```python
from build123d import *

# Parameters (mm, degrees)
SKETCH2_R           = 12.7
SKETCH2_R_2         = 10.6807
BOSS_EXTRUDE1_DEPTH = 19.05
BOSS_EXTRUDE2_REACH = 33.75
SKETCH5_R           = 12.7
CUT_EXTRUDE1_REACH  = 33.75
SKETCH6_R           = 10.6807


with BuildPart() as part:
    # Sketch2 → Boss-Extrude1 (new body, symmetric)
    with BuildSketch(Plane(origin=(0, 0, 0), x_dir=(0, 0, -1), z_dir=(1, 0, 0))):
        Circle(SKETCH2_R)
        Circle(SKETCH2_R_2, mode=Mode.SUBTRACT)
    extrude(amount=BOSS_EXTRUDE1_DEPTH, both=True)

    # Sketch5 → Boss-Extrude2 (add, up to next)
    with BuildSketch(Plane(origin=(0, 19.05, 0), x_dir=(1, 0, 0), z_dir=(0, 1, 0)), mode=Mode.PRIVATE) as boss_extrude2_sk1:
        Circle(SKETCH5_R)
    boss_extrude2_tool1 = extrude(boss_extrude2_sk1.sketch, amount=-BOSS_EXTRUDE2_REACH, mode=Mode.PRIVATE) - part.part
    add(boss_extrude2_tool1.solids().sort_by_distance((0, 19.05, 0))[0])

    # Sketch6 → Cut-Extrude1 (cut, up to next)
    with BuildSketch(Plane(origin=(0, 19.05, 0), x_dir=(1, 0, 0), z_dir=(0, 1, 0)), mode=Mode.PRIVATE) as cut_extrude1_sk1:
        Circle(SKETCH6_R)
    cut_extrude1_tool1 = extrude(cut_extrude1_sk1.sketch, amount=-CUT_EXTRUDE1_REACH, mode=Mode.PRIVATE) & part.part
    add(cut_extrude1_tool1.solids().sort_by_distance((0, 19.05, 0))[0], mode=Mode.SUBTRACT)


solid = part.part
```
Geometry: final body of the model. Coordinates: model frame, mm. A direction names the side the tool comes from. Coordinates: 2 decimals unless noted, no trailing zeros. Loops run counter-clockwise (first coordinate to the right, second up) from the corner with the lowest first, then second, coordinate; pieces in that order, holes last. Notation, with made-up numbers: M 11.25,39.25 L 67.25,39.25 A21 cw 67.25,64.25 Z; hole C 49.25,-17.75 d2. An arc over 180 degrees is marked long. Put each result on its own line as item: value.
(1) Access query for faces 1 (the face through (-0.267, -10.427, 2.315)), 2 (the face through (0.27, -12.4, 2.75)). Directions: +Z, -Z, +X, -X, +Y, -Y. A direction counts if a zero-diameter tool reaches every point of the face in a straight line with its end or side. Return the directions, or none.
Answer sheet:
face 1: +X, -X
face 2: none
(2) Cut plane D-D on z = 7. Return the cut outline in (x, y), then the cut area to 3 significant figures.
Answer sheet:
outline: M -19.05,-10.6 L 19.05,-10.6 L 19.05,-8.07 L -19.05,-8.07 Z; M -19.05,8.07 L -8.07,8.07 L -8.07,19.05 L -10.6,19.05 L -10.6,10.6 L -19.05,10.6 Z; M 8.07,8.07 L 19.05,8.07 L 19.05,10.6 L 10.6,10.6 L 10.6,19.05 L 8.07,19.05 Z
area: 195 mm^2
(3) First-contact query: pin 1 (3 mm diameter, centred on x = 4.5, z = -6.5, fed in from -Y); pin 2 (2 mm diameter, centred on x = 13.5, z = -5, fed in from -Y); pin 3 (2 mm diameter, centred on x = -6, y = -4, fed in from +Z); pin 4 (12 mm diameter, centred on y = 1.5, z = -2.5, fed in from -X). Flat tips, straight axial feed; report the tip coordinate or a pass-through.
Answer sheet:
pin 1: stops at y = -11.67
pin 2: stops at y = -12.05
pin 3: stops at z = 12.34
pin 4: passes through
(4) Cut plane B-B on y = -3. Return the cut outline in (x, z).
Answer sheet:
outline: M -19.05,-12.34 L 19.05,-12.34 L 19.05,-10.25 L -19.05,-10.25 Z; M -19.05,10.25 L 19.05,10.25 L 19.05,12.34 L -19.05,12.34 Z
(5) Material intervals for probe 1 along Z at (x, y) = (0, 11.75); probe 2 along X at (y, z) = (11, 0); probe 3 along Z at (x, y) = (10.5, -8), sorted ascending.
Answer sheet:
probe 1: z = -12.7 to -10.68, 10.68 to 12.7
probe 2: x = -19.05 to -10.68, 10.68 to 19.05
probe 3: z = -9.86 to -7.08, 7.08 to 9.86
(6) Draft query along X for faces 3 (the face through (-1.653, 13.892, -12.592)), 4 (the face through (19.05, 9, 7)), 5 (the face through (-2.315, 11.775, 10.427)), 6 (the face through (-7, 19.05, -9)). Return one class per face: pulls with the +X half, pulls with the -X half, needs draft (parallel to the pull), parting line crosses it, or undercut.
Answer sheet:
face 3: parting line crosses it
face 4: pulls with the +X half
face 5: undercut
face 6: needs draft
(7) Cut plane C-C on x = 0. Return the cut outline in (y, z).
Answer sheet:
outline: M 0,-12.7 L 19.05,-12.7 L 19.05,-10.68 L 0,-10.68 A10.68 cw 0,10.68 L 19.05,10.68 L 19.05,12.7 L 0,12.7 A12.7 ccw Z
(8) Cut plane A-A on z = 0. Return the cut outline in (x, y), then the cut area to 3 significant figures.
Answer sheet:
outline: M -19.05,-12.7 L 19.05,-12.7 L 19.05,-10.68 L -19.05,-10.68 Z; M -19.05,10.68 L -10.68,10.68 L -10.68,19.05 L -12.7,19.05 L -12.7,12.7 L -19.05,12.7 Z; M 10.68,10.68 L 19.05,10.68 L 19.05,12.7 L 12.7,12.7 L 12.7,19.05 L 10.68,19.05 Z
area: 136 mm^2
